For this review, take the finished solid that the model builds, in its own axes (mm). A direction names the side the tool comes from. Give positions to 0.01 mm unless a question says otherwise; leave off trailing zeros. Loops run counter-clockwise (first coordinate to the right, second up) from the corner with the lowest first, then second, coordinate; pieces in that order, holes last. Notation, with made-up numbers: (16, -5) - (20, -5) arc R22 ccw to (20, 24) - close; hole circle Ø3 at (19, 79.5). An arc over 180 degrees is marked (long way). Answer in a Markdown table with one row per item.
```python
from build123d import *

# Parameters (mm, degrees)
BOSS_EXTRUDE1_DEPTH = 145
SKETCH2_R           = 30
CUT_EXTRUDE1_DEPTH  = 180.652442232
SKETCH3_R           = 5
CUT_EXTRUDE2_DEPTH  = 10


with BuildPart() as part:
    # Sketch1 → Boss-Extrude1 (new body)
    with BuildSketch(Plane.XY):
        Polygon((0, -37.5), (0, 37.5), (75, 37.5), (75, 31.15), (6.35, 31.15), (6.35, -31.15), (75, -31.15), (75, -37.5), align=None)
    extrude(amount=BOSS_EXTRUDE1_DEPTH)

    # Sketch2 → Cut-Extrude1 (cut, through all)
    with BuildSketch(Plane(origin=(0, 37.5, 0), x_dir=(1, 0, 0), z_dir=(0, 1, 0))):
        with Locations(Location((40, -72.5, 0), (0, 0, 270))):
            Circle(SKETCH2_R)
    extrude(amount=-CUT_EXTRUDE1_DEPTH, mode=Mode.SUBTRACT)

    # Sketch3 → Cut-Extrude2 (cut)
    with BuildSketch(Plane(origin=(6.35, 0, 0), x_dir=(0, 0, -1), z_dir=(1, 0, 0))):
        with Locations((-107.5, 0)):
            Circle(SKETCH3_R)
        with Locations((-37.5, 0)):
            Circle(SKETCH3_R)
    extrude(amount=-CUT_EXTRUDE2_DEPTH, mode=Mode.SUBTRACT)


solid = part.part
```
1. We need section D-D, the plane z = 72.5. Give the boundary of the cut face in (x, y), and give its area (3 significant figures).
Values:
| item | result |
|---|---|
| outline | (0, -37.5) - (10, -37.5) - (10, -31.15) - (6.35, -31.15) - (6.35, 31.15) - (10, 31.15) - (10, 37.5) - (0, 37.5) - close; (70, -37.5) - (75, -37.5) - (75, -31.15) - (70, -31.15) - close; (70, 31.15) - (75, 31.15) - (75, 37.5) - (70, 37.5) - close |
| area | 586 mm^2 |
2. Mouldability with a two-part tool opening along Y and no side actions: class faces 1 (the face through (4, -5, 0)), 2 (the face through (12, 37.5, 55)), 3 (the face through (9.7, -31.15, 71.5)) as released by +Y, released by -Y, zero draft, split by the parting line, or undercut.
Values:
| item | result |
|---|---|
| face 1 | zero draft |
| face 2 | released by +Y |
| face 3 | undercut |
3. We need section A-A, the plane z = 37.5. Give the boundary of the cut face in (x, y).
Values:
| item | result |
|---|---|
| outline | (0, -37.5) - (75, -37.5) - (75, -31.15) - (6.35, -31.15) - (6.35, -5) - (0, -5) - close; (0, 5) - (6.35, 5) - (6.35, 31.15) - (75, 31.15) - (75, 37.5) - (0, 37.5) - close |
4. For faces 4 (the face through (72, 31.15, 71)), 5 (the face through (3.219, 0.22, 42.495)), list the 3-axis set-ups (+Z, -Z, +X, -X, +Y, -Y) from which the entire face can be reached by the end or side of a thin tool; tool diameter is ignored.
Values:
| item | result |
|---|---|
| face 4 | +Z, -Z, +X |
| face 5 | +X, -X |
5. Wall thickness on line 1 (Y direction, x = 34.5, z = 31.5); line 2 (X direction, y = 32.5, z = 72.5); line 3 (Y direction, x = 3.5, z = 37.5): over which ranges is each line inside the solid? List them lowest first. Write a range as [from, to].
Values:
| item | result |
|---|---|
| line 1 | y = [-37.5, -31.15], [31.15, 37.5] |
| line 2 | x = [0, 10], [70, 75] |
| line 3 | y = [-37.5, -5], [5, 37.5] |
6. Clearance check with flat-ended pins moving along their axes: pin 1 (3 mm diameter, centred on x = 12.5, y = -28, fed in from -Z); pin 2 (10 mm diameter, centred on y = 1.5, z = 70.5, fed in from +X). State where each tip first meets the part, or that it passes through.
Values:
| item | result |
|---|---|
| pin 1 | passes through |
| pin 2 | stops at x = 6.35 |
7. We need section C-C, the plane y = 0. Give the boundary of the cut face in (x, z).
Values:
| item | result |
|---|---|
| outline | (0, 0) - (6.35, 0) - (6.35, 32.5) - (0, 32.5) - close; (0, 42.5) - (6.35, 42.5) - (6.35, 102.5) - (0, 102.5) - close; (0, 112.5) - (6.35, 112.5) - (6.35, 145) - (0, 145) - close |
8. We need section B-B, the plane x = 40. Give the boundary of the cut face in (y, z).
Values:
| item | result |
|---|---|
| outline | (-37.5, 0) - (-31.15, 0) - (-31.15, 42.5) - (-37.5, 42.5) - close; (-37.5, 102.5) - (-31.15, 102.5) - (-31.15, 145) - (-37.5, 145) - close; (31.15, 0) - (37.5, 0) - (37.5, 42.5) - (31.15, 42.5) - close; (31.15, 102.5) - (37.5, 102.5) - (37.5, 145) - (31.15, 145) - close |
